Could you check a few things on this model? Use its own coordinates, in mm. Round coordinates to 2 decimals unless told otherwise and drop trailing zeros. Write each loop counter-clockwise with the first axis right and the second up, starting at its lowest first coordinate (ties: lowest second). Pieces come first, ordered by that corner, then holes. Notation, with made-up numbers: (39.5, 68) -> (50.5, 68) arc R20 ccw to (50.5, 86) -> close; hole circle Ø11 at (-13, 22.25). An arc over 180 degrees is marked (long way). Answer as CSV lines item,"result". Start each with the question number.
Q1. If I drill on line 1 (X direction, y = -2.9, z = -9); line 2 (Z direction, x = 185, y = -1.35), over which ranges is the centre line in solid material (lowest first)? Write a range as [from, to].
Q2. Imagine slicing it at C-C on x = 89.5. Please give me the cut outline in (y, z) (3 decimals), and give its area (3 significant figures).
Q3. Imagine slicing it at B-B on y = -1.1. Please give me the cut outline in (x, z), and give its area (3 significant figures).
Q4. Imagine slicing it at A-A on z = -63. Please give me the cut outline in (x, y) (3 decimals).
from build123d import *

# Parameters (mm, degrees)
F0_W          = 551.280781
F0_H          = 595.958948
F2_DEPTH      = 3.175
F1_W          = 391.17673
F1_H          = 113.006599
F3_DEPTH      = 25.4
F3_DEPTH_BACK = 25.4


with BuildPart() as f2:
    # F0 (on Front) → F2 (new body)
    with BuildSketch(Plane.XZ):
        with Locations((183.218337, 187.043697)):
            Rectangle(F0_W, F0_H)
    extrude(amount=F2_DEPTH)

    # F1 (on face) → F3 (cut, two sides)
    with BuildSketch(Plane.XZ) as f3_sk:
        with Locations((181.670889, -52.791416)):
            Rectangle(F1_W, F1_H)
    extrude(amount=F3_DEPTH, mode=Mode.SUBTRACT)
    extrude(f3_sk.sketch, amount=-F3_DEPTH_BACK, mode=Mode.SUBTRACT)


solid = f2.part
Checks:
1,line 1,"[-92.42, -13.92], [377.26, 458.86]"
1,line 2,"[-110.94, -109.29], [3.71, 485.02]"
2,outline,"(-3.175, -110.936) -> (0, -110.936) -> (0, -109.295) -> (-3.175, -109.295) -> close; (-3.175, 3.712) -> (0, 3.712) -> (0, 485.023) -> (-3.175, 485.023) -> close"
2,area,"1,530 mm^2"
3,outline,"(-92.42, -110.94) -> (458.86, -110.94) -> (458.86, 485.02) -> (-92.42, 485.02) -> close; hole (-13.92, -109.29) -> (377.26, -109.29) -> (377.26, 3.71) -> (-13.92, 3.71) -> close"
3,area,"284,000 mm^2"
4,outline,"(-92.422, -3.175) -> (-13.917, -3.175) -> (-13.917, 0) -> (-92.422, 0) -> close; (377.259, -3.175) -> (458.859, -3.175) -> (458.859, 0) -> (377.259, 0) -> close"
